Verification items for this drawing (mm, ordinates from the low corner). Coordinates: 2 decimals unless noted, no trailing zeros. Loops run counter-clockwise (first coordinate to the right, second up) from the corner with the lowest first, then second, coordinate; pieces in that order, holes last. Notation, with made-up numbers: M -9,39 L -1,39 A29 ccw -1,78 Z; hole C -12.75,-12 d2. An arc over 180 degrees is marked long. Use CSV: the item, a comma, the result in double quotes.
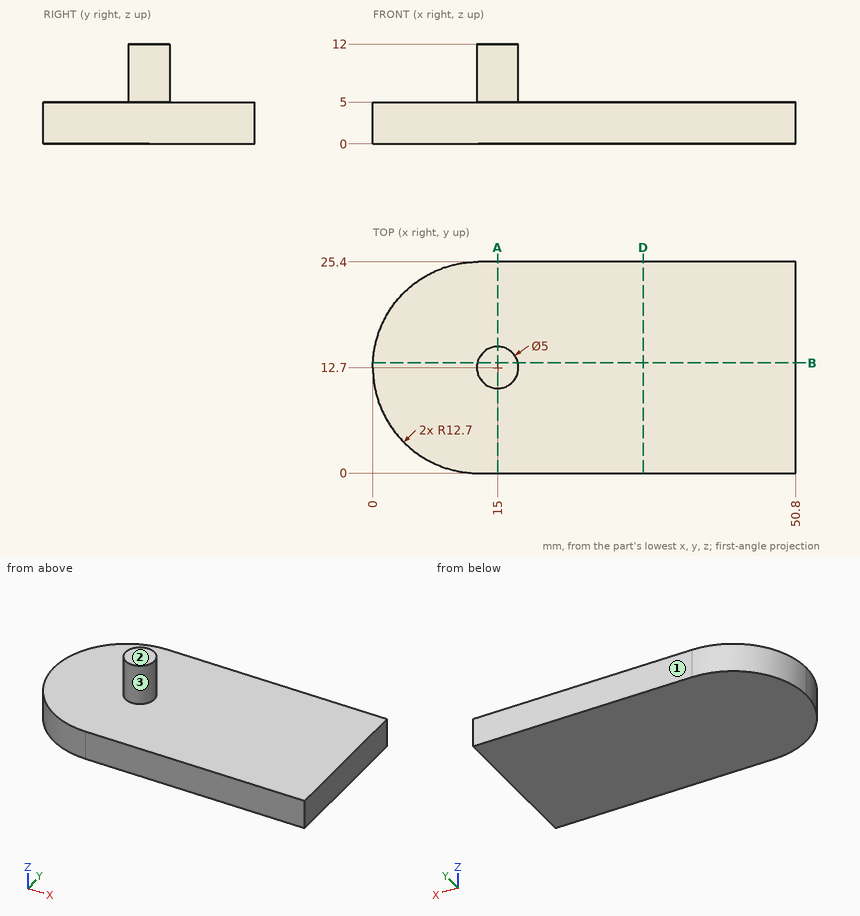
1. Section check D-D, the plane x = 32.5. Record the cut outline in (y, z).
The answers:
outline,"M 0,0 L 25.4,0 L 25.4,5 L 0,5 Z"
2. Thickness scan on line 1 (X direction, y = 12.5, z = 10.5); line 2 (Z direction, x = 36, y = 14); line 3 (X direction, y = 23.75, z = 3). Record the ranges inside material, lowest first. Write a range as [from, to].
The answers:
line 1,"[12.51, 17.49]"
line 2,"[0, 5]"
line 3,"[6.44, 50.8]"
3. Gauge pin test, flat ends, axial feed: P1, Ø1.5, axis at y = 11.5, z = 10, coming from the +X side; P2, Ø4, axis at x = 19, z = 7.5, coming from the +Y side; P3, Ø8, axis at x = 8, y = 22, coming from the +Z side. Record the tip position at first contact, or that the pin passes through.
The answers:
P1,"x = 17.46"
P2,"y = 14.2"
P3,"z = 5"
4. Release check for a two-part mould opening along Y. For the marked faces 1, 2 and 3 record: +Y half, -Y half, draft (parallel to the pull), parting line (faces both ways), or undercut.
The answers:
face 1,"+Y half"
face 2,"draft"
face 3,"parting line"
5. Section check A-A, the plane x = 15. Record the cut outline in (y, z), plus the area to 3 significant figures.
The answers:
outline,"M 0,0 L 25.4,0 L 25.4,5 L 15.2,5 L 15.2,12 L 10.2,12 L 10.2,5 L 0,5 Z"
area,"162 mm^2"
6. Section check B-B, the plane y = 13.25. Record the cut outline in (x, z), plus the area to 3 significant figures.
The answers:
outline,"M 0.01,0 L 50.8,0 L 50.8,5 L 17.44,5 L 17.44,12 L 12.56,12 L 12.56,5 L 0.01,5 Z"
area,"288 mm^2"
